Can you work these out from the drawing? Everything is in mm from the part's minimum corner. A direction names the side the tool comes from. Coordinates: 2 decimals unless noted, no trailing zeros. Order: outer loops, then holes, each group sorted by start corner. A loop starts at its lowest first (then second) coordinate and runs counter-clockwise, first axis right, second up. Notation, with made-up numbers: (-23, -19.5) -> (30, -19.5) arc R22 cw to (30, -13.5) -> close; hole circle Ø7 at (11.5, -17). An arc over 180 degrees is marked (long way). Put each result on its own line as item: value. Start each with the question number.
Q1. Will these pins go through, and if not, where does the flat tip stop? pin 1 (8 mm diameter, centred on y = 8, z = 25, fed in from +X); pin 2 (8 mm diameter, centred on y = 7, z = 24.5, fed in from -X); pin 3 (6.5 mm diameter, centred on x = 24.5, y = 7.5, fed in from -Z).
Q2. If we section it at C-C (z = 25): Please give me the cut outline in (x, y), and give its area (3 significant figures).
Q3. If we section it at A-A (z = 20.5): Please give me the cut outline in (x, y).
Q4. If we section it at D-D (y = 9.75): Count the separate pieces of the cut face and the enclosed holes in it, and give its area (3 significant figures).
Q5. We'd pull the mould along Y, two halves only. Please class the marked faces 5, 6 and 7: +Y half, -Y half, draft (parallel to the pull), parting line (faces both ways), or undercut.
Q6. For the marked faces 1, 2, 3 and 4, which set-ups out of +Z, -Z, +X, -X, +Y, -Y let a thin tool reach every point of the face, with its end or its side?
Q7. If we section it at B-B (x = 19.5): Please give me the cut outline in (y, z).
Q8. Please list where these lines run through material, in increasing order: line 1 along Y through (x, z) = (17, 25); line 2 along X through (y, z) = (15, 19); line 3 along X through (y, z) = (4.5, 13).
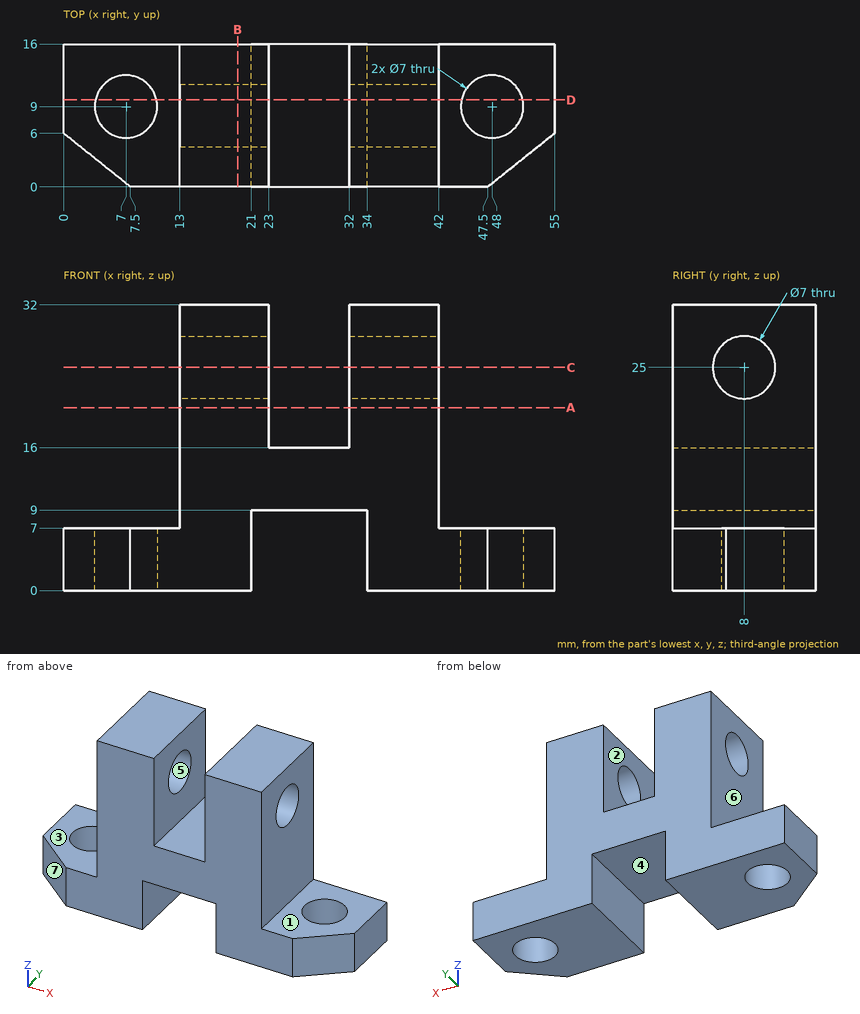
The answers:
1. pin 1: x = 42
1. pin 2: x = 13
1. pin 3: z = 9
2. outline: (13, 0) -> (23, 0) -> (23, 4.5) -> (13, 4.5) -> close; (13, 11.5) -> (23, 11.5) -> (23, 16) -> (13, 16) -> close; (32, 0) -> (42, 0) -> (42, 4.5) -> (32, 4.5) -> close; (32, 11.5) -> (42, 11.5) -> (42, 16) -> (32, 16) -> close
2. area: 180 mm^2
3. outline: (13, 0) -> (23, 0) -> (23, 16) -> (13, 16) -> close; (32, 0) -> (42, 0) -> (42, 16) -> (32, 16) -> close
4. separate pieces: 5
4. enclosed holes: 0
4. area: 632 mm^2
5. face 5: undercut
5. face 6: draft
5. face 7: -Y half
6. face 1: +Z, +X, +Y, -Y
6. face 2: +Z, +Y, -Y
6. face 3: +Z, -X, +Y, -Y
6. face 4: -Z, +Y, -Y
7. outline: (0, 0) -> (16, 0) -> (16, 32) -> (0, 32) -> close; hole circle Ø7 at (8, 25)
8. line 1: 0 to 4.5, 11.5 to 16
8. line 2: 13 to 23, 32 to 42
8. line 3: 13 to 42
